Can you work these out from the model? Positions are in its coordinate system, mm. Face numbers are marked on the shaded views. A direction names the side the tool comes from. Round coordinates to 2 decimals unless told otherwise and drop trailing zeros. Order: outer loops, then holes, each group sorted by start corner. A loop starts at its lowest first (then second) coordinate and runs counter-clockwise, first axis right, second up. Notation, with made-up numbers: (-22, -36.5) - (-18, -36.5) arc R14 cw to (-18, -22.5) - close; hole circle Ø9 at (-39, -27.5). An arc over 180 degrees is marked (long way). Write item = value, one per line.
from build123d import *

# Parameters (mm, degrees)
SKETCH1_W           = 70
SKETCH1_H           = 40
BOSS_EXTRUDE1_DEPTH = 10
SKETCH2_R           = 1.65
CUT_EXTRUDE1_DEPTH  = 11
FILLET1_R           = 10
SHELL2_T            = -1
SKETCH3_R           = 2.65
SKETCH3_R_2         = 1.65
BOSS_EXTRUDE2_DEPTH = 4
CUT_EXTRUDE2_DEPTH  = 2


with BuildPart() as part:
    # Sketch1 → Boss-Extrude1 (new body)
    with BuildSketch(Plane.XY):
        Rectangle(SKETCH1_W, SKETCH1_H)
    extrude(amount=BOSS_EXTRUDE1_DEPTH)

    # Sketch2 → Cut-Extrude1 (cut, through all)
    with BuildSketch(Plane(origin=(0, 0, 0), x_dir=(-1, 0, 0), z_dir=(0, 0, -1))):
        with Locations((-25, 0)):
            Circle(SKETCH2_R)
        with Locations((-2, 0)):
            Circle(SKETCH2_R)
        with Locations((19, -1)):
            Circle(SKETCH2_R)
    extrude(amount=-CUT_EXTRUDE1_DEPTH, mode=Mode.SUBTRACT)

    # Fillet1
    fillet1_edges = [part.edges().sort_by_distance(p)[0] for p in [
        (35, -20, 5),
        (-35, -20, 5),
        (-35, 20, 5),
        (35, 20, 5),
    ]]
    fillet(fillet1_edges, radius=FILLET1_R)

    # Shell2
    shell2_openings = [part.faces().sort_by_distance(p)[0] for p in [
        (23.35, 0, 0),
    ]]
    offset(amount=SHELL2_T, openings=shell2_openings, kind=Kind.INTERSECTION)

    # Sketch3 → Boss-Extrude2 (add)
    with BuildSketch(Plane(origin=(0, 0, 0), x_dir=(-1, 0, 0), z_dir=(0, 0, -1))):
        with Locations((-2, 0)):
            Circle(SKETCH3_R)
        with Locations((-2, 0)):
            Circle(SKETCH3_R_2, mode=Mode.SUBTRACT)
        with Locations((-25, 0)):
            Circle(SKETCH3_R)
        with Locations((-25, 0)):
            Circle(SKETCH3_R_2, mode=Mode.SUBTRACT)
    extrude(amount=BOSS_EXTRUDE2_DEPTH)

    # Sketch4 → Cut-Extrude2 (cut)
    with BuildSketch(Plane(origin=(0, 0, 0), x_dir=(-1, 0, 0), z_dir=(0, 0, -1))):
        with BuildLine():
            Line((35, -10), (35, 10))
            ThreePointArc((35, 10), (32.071067812, 17.071067812), (25, 20))
            Line((25, 20), (-25, 20))
            ThreePointArc((-25, 20), (-32.071067812, 17.071067812), (-35, 10))
            Line((-35, 10), (-35, -10))
            ThreePointArc((-35, -10), (-32.071067812, -17.071067812), (-25, -20))
            Line((-25, -20), (25, -20))
            ThreePointArc((25, -20), (32.071067812, -17.071067812), (35, -10))
        make_face()
        with BuildLine():
            Line((33, -10), (33, 10))
            ThreePointArc((33, 10), (30.656854249, 15.656854249), (25, 18))
            Line((25, 18), (-25, 18))
            ThreePointArc((-25, 18), (-30.656854249, 15.656854249), (-33, 10))
            Line((-33, 10), (-33, -10))
            ThreePointArc((-33, -10), (-30.656854249, -15.656854249), (-25, -18))
            Line((-25, -18), (25, -18))
            ThreePointArc((25, -18), (30.656854249, -15.656854249), (33, -10))
        make_face(mode=Mode.SUBTRACT)
    extrude(amount=-CUT_EXTRUDE2_DEPTH, mode=Mode.SUBTRACT)


solid = part.part
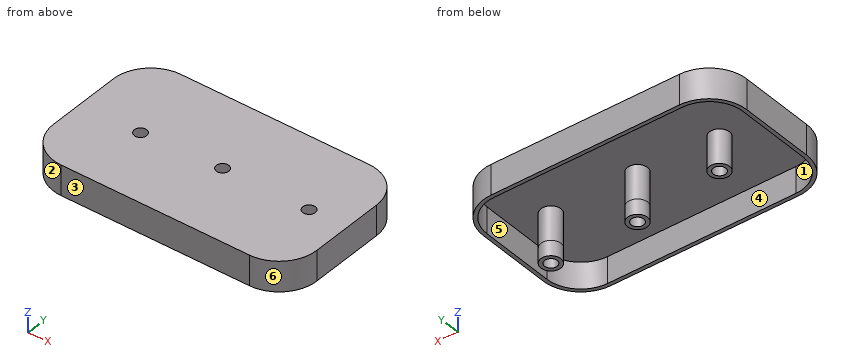
(1) If we section it at B-B (z = 5.75): Write out the boundary of the cut face in (x, y), plus the area to 3 significant figures.
Computed:
outline = (-35, -10) arc R10 ccw to (-25, -20) - (25, -20) arc R10 ccw to (35, -10) - (35, 10) arc R10 ccw to (25, 20) - (-25, 20) arc R10 ccw to (-35, 10) - close; circle Ø5.3 at (-19, -1); circle Ø5.3 at (2, 0); circle Ø5.3 at (25, 0); hole (-34, -10) arc R9 ccw to (-25, -19) - (25, -19) arc R9 ccw to (34, -10) - (34, 10) arc R9 ccw to (25, 19) - (-25, 19) arc R9 ccw to (-34, 10) - close; hole circle Ø3.3 at (-19, -1); hole circle Ø3.3 at (2, 0); hole circle Ø3.3 at (25, 0)
area = 240 mm^2
(2) If we section it at D-D (z = -1): Write out the boundary of the cut face in (x, y).
Computed:
outline = circle Ø5.3 at (2, 0); circle Ø5.3 at (25, 0); hole circle Ø3.3 at (2, 0); hole circle Ø3.3 at (25, 0)
(3) Will these pins go through, and if not, where does the flat tip stop? P1, Ø2.5, axis at x = 25, y = 0, coming from the +Z side; P2, Ø1, axis at x = -8.5, y = 7.5, coming from the -Z side; P3, Ø10, axis at x = -2, y = 15, coming from the -Z side; P4, Ø2.5, axis at x = -20.5, y = 0, coming from the -Z side.
Computed:
P1 = through
P2 = 9
P3 = 2
P4 = 0
(4) If we section it at A-A (x = -19): Write out the boundary of the cut face in (y, z).
Computed:
outline = (-20, 2) - (-19, 2) - (-19, 9) - (-3.65, 9) - (-3.65, 0) - (-2.65, 0) - (-2.65, 10) - (-20, 10) - close; (0.65, 0) - (1.65, 0) - (1.65, 9) - (19, 9) - (19, 2) - (20, 2) - (20, 10) - (0.65, 10) - close
(5) Thinking about a two-plate mould opening in X: for the marked faces 1, 2, 3 and 4, which applies, +X half, -X half, draft (parallel to the pull), parting line (faces both ways), or undercut?
Computed:
face_1 = undercut
face_2 = -X half
face_3 = draft
face_4 = undercut
(6) If we section it at C-C (x = 2): Write out the boundary of the cut face in (y, z), plus the area to 3 significant figures.
Computed:
outline = (-20, 2) - (-19, 2) - (-19, 9) - (-2.65, 9) - (-2.65, -4) - (-1.65, -4) - (-1.65, 10) - (-20, 10) - close; (1.65, -4) - (2.65, -4) - (2.65, 9) - (19, 9) - (19, 2) - (20, 2) - (20, 10) - (1.65, 10) - close
area = 76.7 mm^2
(7) On a 3-axis mill with a long thin cutter (end or side, diameter ignored), from which of +Z, -Z, +X, -X, +Y, -Y can I reach the whole of each face in a straight line? I mean the marked faces 5 and 6. Say none if no direction works.
Computed:
face_5 = -Z
face_6 = +Z, -Z, +X, -Y
(8) If I drill on line 1 (Y direction, x = -19, z = 3); line 2 (Y direction, x = 25, z = 7); line 3 (Y direction, x = -2.5, z = 5.5), over which ranges is the centre line in solid material (lowest first)? Write a range as from..to.
Computed:
line_1 = -20..-19, -3.65..-2.65, 0.65..1.65, 19..20
line_2 = -20..-19, -2.65..-1.65, 1.65..2.65, 19..20
line_3 = -20..-19, 19..20
